Here's the drawing with two shaded views (mm, measured from the low corner). I have some questions. Give positions to 0.01 mm unless a question says otherwise; leave off trailing zeros. Write each loop counter-clockwise with the first axis right and the second up, starting at its lowest first coordinate (ties: lowest second). Pieces come first, ordered by that corner, then holes.
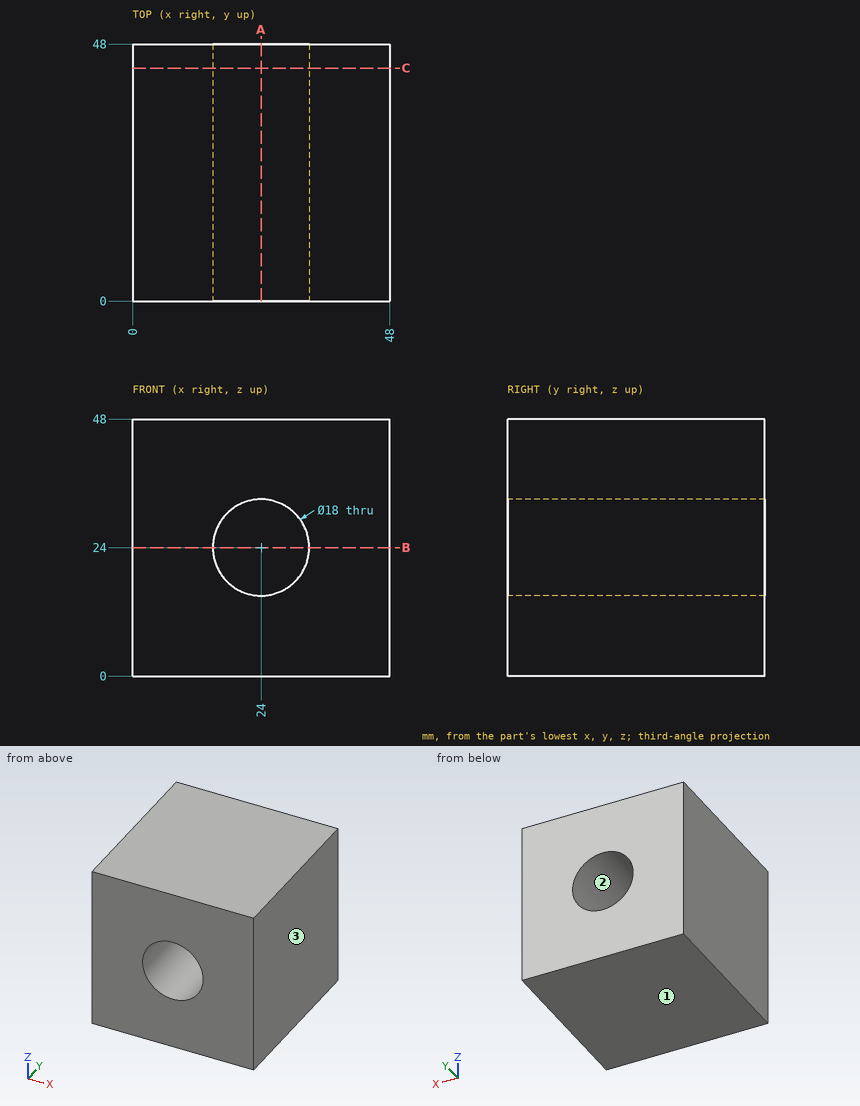
1) Please list where these lines run through material, in increasing order: L1, parallel to Z at x = 24, y = 31.5; L2, parallel to X at y = 18, z = 23.5; L3, parallel to X at y = 24.5, z = 21.
Values follow:
L1: z = 0 to 15, 33 to 48
L2: x = 0 to 15.01, 32.99 to 48
L3: x = 0 to 15.51, 32.49 to 48
2) Suppose I cut it at B-B on z = 24. Write out the boundary of the cut face in (x, y), plus the area to 3 significant figures.
Values follow:
outline: (0, 0) - (15, 0) - (15, 48) - (0, 48) - close; (33, 0) - (48, 0) - (48, 48) - (33, 48) - close
area: 1,440 mm2
3) If we mould it in two halves opening along X, with no side actions, what happens to the marked faces 1, 2 and 3? For each: +X half, -X half, draft (parallel to the pull), parting line (faces both ways), or undercut.
Values follow:
face 1: draft
face 2: undercut
face 3: +X half
4) Suppose I cut it at A-A on x = 24. Write out the boundary of the cut face in (y, z), plus the area to 3 significant figures.
Values follow:
outline: (0, 0) - (48, 0) - (48, 15) - (0, 15) - close; (0, 33) - (48, 33) - (48, 48) - (0, 48) - close
area: 1,440 mm2
5) Suppose I cut it at C-C on y = 43.5. Write out the boundary of the cut face in (x, z), plus the area to 3 significant figures.
Values follow:
outline: (0, 0) - (48, 0) - (48, 48) - (0, 48) - close; hole circle Ø18 at (24, 24)
area: 2,050 mm2
